```python
from build123d import *

# Parameters (mm, degrees)
F0_W      = 51
F0_H      = 84
F0_R      = 1.75
F1_DEPTH  = 1.7
F2_W      = 9.4
F2_H      = 16
F3_DEPTH  = 12
F4_R      = 3.5
F5_DEPTH  = 19
F6_R      = 6.5
F7_DEPTH  = 22
F8_W      = 30
F8_H      = 7.5
F9_DEPTH  = 10
F10_R     = 5.9425868451
F10_R_2   = 3
F11_DEPTH = 15


with BuildPart() as f1:
    # F0 (on Top) → F1 (new body)
    with BuildSketch(Plane.XY):
        Rectangle(F0_W, F0_H)
        with Locations((-22, -38.5)):
            Circle(F0_R, mode=Mode.SUBTRACT)
        with Locations((22, -38.5)):
            Circle(F0_R, mode=Mode.SUBTRACT)
        with Locations((-22, 38.5)):
            Circle(F0_R, mode=Mode.SUBTRACT)
        with Locations((22, 38.5)):
            Circle(F0_R, mode=Mode.SUBTRACT)
    extrude(amount=F1_DEPTH)

    # F2 (on face) → F3 (join)
    with BuildSketch(Plane.XY.offset(1.7)):
        with Locations((13.1, -34)):
            Rectangle(F2_W, F2_H)
    extrude(amount=F3_DEPTH)

    # F4 (on face) → F5 (join)
    with BuildSketch(Plane.XZ.offset(42)):
        with Locations((13.1, 7.7)):
            Circle(F4_R)
    extrude(amount=F5_DEPTH)

    # F6 (on face) → F7 (join)
    with BuildSketch(Plane.XY.offset(1.7)):
        with Locations((17.1509794891, -10.8471838757)):
            Circle(F6_R)
        with Locations((-16.6441705078, -10.8471838757)):
            Circle(F6_R)
    extrude(amount=F7_DEPTH)

    # F8 (on face) → F9 (join)
    with BuildSketch(Plane.XY.offset(1.7)):
        with Locations((0, 38.25)):
            Rectangle(F8_W, F8_H)
    extrude(amount=F9_DEPTH)

    # F10 (on face) → F11 (cut)
    with BuildSketch(Plane.XZ.offset(61)):
        with Locations((13.1, 7.7)):
            Circle(F10_R)
        with Locations((13.1, 7.7)):
            Circle(F10_R_2, mode=Mode.SUBTRACT)
    extrude(amount=-F11_DEPTH, mode=Mode.SUBTRACT)


solid = f1.part
```
Geometry check sheet. Reference: the model listing, model coordinates, mm. A direction names the side the tool comes from. Give positions to 0.01 mm unless a question says otherwise; leave off trailing zeros. Order: outer loops, then holes, each group sorted by start corner. A loop starts at its lowest first (then second) coordinate and runs counter-clockwise, first axis right, second up. Notation, with made-up numbers: (5, 25) - (46, 25) arc R26 ccw to (46, 63) - close; hole circle Ø4 at (-26, 34.25). An arc over 180 degrees is marked (long way). Write item = value, one per line. Start each with the question number.
1) Draft check along Y on faces 6 (the cylindrical face through (23.155, -13.337, 12.546)), 7 (the cylindrical face through (-23.39, -39.56, 0.84)), 8 (the flat face through (13, -61, 8)), 9 (the flat face through (0, 1, 0)). Enter one of: released by +Y, released by -Y, zero draft, split by the parting line, or undercut.
2) Section check C-C (y = -33). Enter the section's corners in (x, z).
3) Section check B-B (x = 22). Enter the section's corners in (y, z).
4) Gauge pin test, flat ends, axial feed: pin 1 Ø3 at (x, y) = (-22, 38.5) entering from +Z (3 decimals); pin 2 Ø9.5 at (y, z) = (-33.5, 7) entering from -X; pin 3 Ø8 at (y, z) = (37.5, 7.5) entering from +X; pin 4 Ø8 at (x, y) = (7.5, -22.5) entering from +Z. Record the tip position at first contact, or that the pin passes through.
5) Section check D-D (z = 7.7). Enter the section's corners in (x, y).
6) Scan lines: L1, parallel to Y at x = -22, z = 0.9; L2, parallel to Z at x = -4, y = 34; L3, parallel to X at y = -36.5, z = 6. Record each from-to range of solid material in increasing order.
7) Section check A-A (y = 38.5). Enter the section's corners in (x, z).
8) Access from +Z, -Z, +X, -X, +Y, -Y to the whole of each face (thin tool, end or side, straight path). Record for faces 1 (the flat face through (13, -26, 8)), 2 (the flat face through (8.4, -34, 8)), 3 (the flat face through (16, -46, 9)), 4 (the flat face through (0, 38, 11.7)), 5 (the flat face through (13, -34, 13.7)).
Geometry check:
q1.face_6 = undercut
q1.face_7 = undercut
q1.face_8 = released by -Y
q1.face_9 = zero draft
q2.outline = (-25.5, 0) - (25.5, 0) - (25.5, 1.7) - (17.8, 1.7) - (17.8, 13.7) - (8.4, 13.7) - (8.4, 1.7) - (-25.5, 1.7) - close
q3.outline = (-42, 0) - (-40.25, 0) - (-40.25, 1.7) - (-42, 1.7) - close; (-36.75, 0) - (36.75, 0) - (36.75, 1.7) - (-6.52, 1.7) - (-6.52, 23.7) - (-15.18, 23.7) - (-15.18, 1.7) - (-36.75, 1.7) - close; (40.25, 0) - (42, 0) - (42, 1.7) - (40.25, 1.7) - close
q4.pin_1 = through
q4.pin_2 = 8.4
q4.pin_3 = 15
q4.pin_4 = 13.7
q5.outline = circle Ø13 at (-16.64, -10.85); (-15, 34.5) - (15, 34.5) - (15, 42) - (-15, 42) - close; (8.4, -42) - (9.6, -42) - (9.6, -46) - (10.1, -46) - (10.1, -61) - (16.1, -61) - (16.1, -46) - (16.6, -46) - (16.6, -42) - (17.8, -42) - (17.8, -26) - (8.4, -26) - close; circle Ø13 at (17.15, -10.85)
q6.L1 = -42 to -40.25, -36.75 to 36.75, 40.25 to 42
q6.L2 = 0 to 1.7
q6.L3 = 8.4 to 17.8
q7.outline = (-25.5, 0) - (-23.75, 0) - (-23.75, 1.7) - (-25.5, 1.7) - close; (-20.25, 0) - (20.25, 0) - (20.25, 1.7) - (15, 1.7) - (15, 11.7) - (-15, 11.7) - (-15, 1.7) - (-20.25, 1.7) - close; (23.75, 0) - (25.5, 0) - (25.5, 1.7) - (23.75, 1.7) - close
q8.face_1 = +Z, +X, -X
q8.face_2 = +Z, -X, -Y
q8.face_3 = -Y
q8.face_4 = +Z, +X, -X, +Y
q8.face_5 = +Z, +X, -X, -Y
